Print and shaded views of the part. All mm, measured from the part's lowest x, y and z. Round coordinates to 2 decimals unless told otherwise and drop trailing zeros. Loops run counter-clockwise (first coordinate to the right, second up) from the corner with the lowest first, then second, coordinate; pieces in that order, holes last. Notation, with made-up numbers: (7, -37.75) - (12, -37.75) arc R13 cw to (12, -14.75) - close; hole circle Ø5 at (45, 42.25). An arc over 180 degrees is marked (long way). Use one line per item in the form item = value.
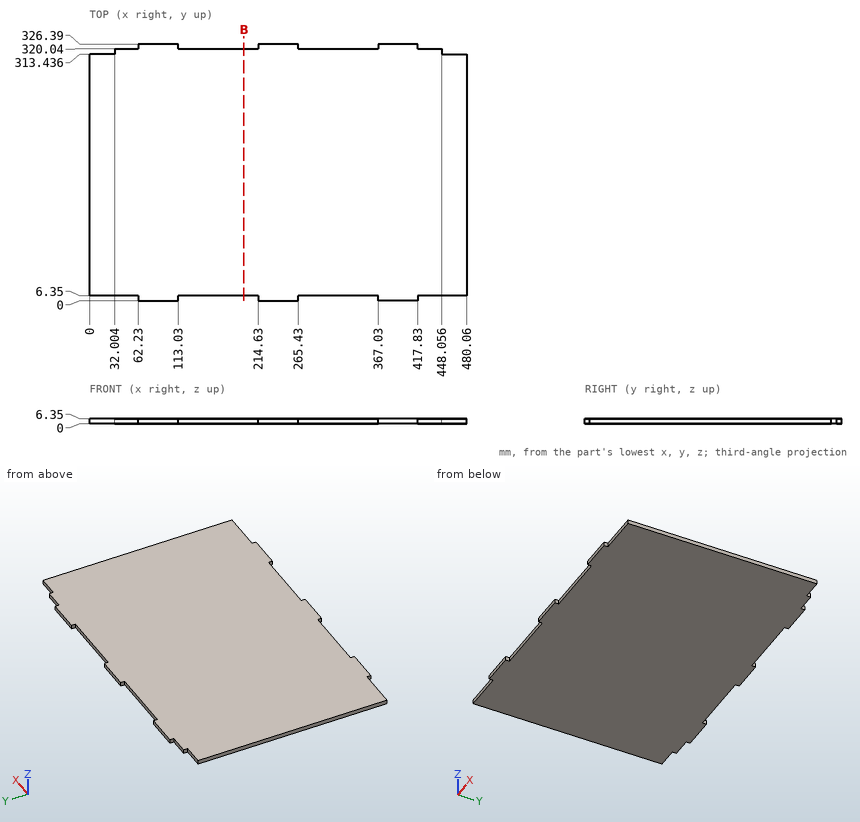
1) Drill centre line: probe 1 along Y at (x, z) = (192, 0.5). Where is it in solid material? Low to high.
Report:
probe_1 = 6.35 to 320.04
2) Flat gauge pins, fed straight in: pin 1 (3 mm diameter, centred on x = 52.5, z = 4, fed in from +Y); pin 2 (3 mm diameter, centred on y = 323, z = 2.5, fed in from -X); pin 3 (12 mm diameter, centred on x = 341.5, y = 177, fed in from -Z); pin 4 (1.9 mm diameter, centred on y = 2.5, z = 2, fed in from +X). Where does each tip first touch, or does it go through?
Report:
pin_1 = 320.04
pin_2 = 62.23
pin_3 = 0
pin_4 = 417.83
3) Slice it at B-B (x = 196.5). Write the cut outline in (y, z).
Report:
outline = (6.35, 0) - (320.04, 0) - (320.04, 6.35) - (6.35, 6.35) - close
